Work out the finished part from the listing and answer in its coordinate system (mm). Face numbers are marked on the shaded views. A direction names the side the tool comes from. Give positions to 0.01 mm unless a question says otherwise; leave off trailing zeros. Write each loop counter-clockwise with the first axis right and the second up, starting at its lowest first coordinate (ties: lowest second). Pieces come first, ordered by that corner, then holes. Notation, with made-up numbers: (3, 21) -> (27, 21) arc R10 ccw to (27, 36) -> close; hole circle Ø6 at (87, -38.75). An arc over 180 degrees is marked (long way). Use a Markdown table: item, result. Add a question column.
Q1. Section A-A, the plane y = 7 is taken. Give the vertices of the cut face in (x, z).
Q2. Section D-D, the plane y = 1 is taken. Give the vertices of the cut face in (x, z).
Q3. For the marked faces 1, 2 and 3, determine the directions among +Z, -Z, +X, -X, +Y, -Y from which every point of the face is accessible in a straight line to the end or side of a thin tool.
Q4. Section C-C, the plane x = 13.35 is taken. Give the vertices of the cut face in (y, z).
Q5. Section B-B, the plane z = -5 is taken. Give the vertices of the cut face in (x, y), plus the area to 3 significant figures.
Q6. Each of these flat-tipped pins is pushed along its axis until it touches: pin 1 Ø2 at (x, z) = (1.5, -6) entering from -Y; pin 2 Ø1.4 at (y, z) = (4.5, 5.5) entering from +X; pin 3 Ø6 at (x, z) = (9.5, -0.5) entering from +Y. Where does it stop, or does it pass through?
Q7. For a pull along Z with two mould halves and no side action, classify the marked faces 4, 5 and 6 as pulls with the +Z half, pulls with the -Z half, needs draft (parallel to the pull), parting line crosses it, or undercut.
Q8. Consider line 1 (X direction, y = 0.3, z = 0); line 2 (Z direction, x = -13.35, y = 0.3); line 3 (X direction, y = 7.25, z = 6.5). Determine where each line is inside the solid, lowest interval first.
from build123d import *

# Parameters (mm, degrees)
SKETCH1_W                = 14.7
SKETCH1_H                = 15
BOSS_EXTRUDE1_DEPTH      = 15.4
SKETCH2_W                = 10.7
SKETCH2_H                = 14.684086862
CUT_EXTRUDE1_DEPTH       = 13
SKETCH4_W                = 2.7
SKETCH4_H                = 3.8
BOSS_EXTRUDE2_DEPTH      = 3
SKETCH5_W                = 10
SKETCH5_H                = 13.4
CUT_EXTRUDE2_DEPTH       = 23.572106681
SKETCH6_W                = 9.3
SKETCH6_H                = 3.8
SKETCH6_H_2              = 2.4
CUT_EXTRUDE3_DEPTH       = 23.719650085
BOSS_EXTRUDE3_DEPTH      = 12
BOSS_EXTRUDE3_DEPTH_BACK = 2.7
SKETCH7_W                = 15
SKETCH7_H                = 2
BOSS_EXTRUDE4_DEPTH      = 12
BOSS_EXTRUDE4_DEPTH_BACK = 2.7
SKETCH8_W                = 15
SKETCH8_H                = 2


with BuildPart() as part:
    # Sketch1 → Boss-Extrude1 (new body)
    with BuildSketch(Plane(origin=(0, 0, 0), x_dir=(1, 0, 0), z_dir=(0, 1, 0))):
        Rectangle(SKETCH1_W, SKETCH1_H)
    extrude(amount=BOSS_EXTRUDE1_DEPTH)

    # Sketch2 → Cut-Extrude1 (cut)
    with BuildSketch(Plane.XY.offset(7.5)):
        with Locations((0, 6.057956569)):
            Rectangle(SKETCH2_W, SKETCH2_H)
    extrude(amount=-CUT_EXTRUDE1_DEPTH, mode=Mode.SUBTRACT)

    # Sketch4 → Boss-Extrude2 (add)
    with BuildSketch(Plane.XY.offset(7.5)):
        with Locations((-6, 7.4)):
            Rectangle(SKETCH4_W, SKETCH4_H)
        with Locations((-6, 12.9)):
            Rectangle(SKETCH4_W, SKETCH4_H)
        with Locations((6, 12.9)):
            Rectangle(SKETCH4_W, SKETCH4_H)
        with Locations((6, 7.4)):
            Rectangle(SKETCH4_W, SKETCH4_H)
        with Locations((-6, 1.9)):
            Rectangle(SKETCH4_W, SKETCH4_H)
        with Locations((6, 1.9)):
            Rectangle(SKETCH4_W, SKETCH4_H)
    extrude(amount=-BOSS_EXTRUDE2_DEPTH)

    # Sketch5 → Cut-Extrude2 (cut, through all)
    with BuildSketch(Plane(origin=(7.35, 0, 0), x_dir=(0, 0, -1), z_dir=(1, 0, 0))):
        with Locations((0.5, 8.7)):
            Rectangle(SKETCH5_W, SKETCH5_H)
    extrude(amount=-CUT_EXTRUDE2_DEPTH, mode=Mode.SUBTRACT)

    # Sketch6 → Cut-Extrude3 (cut, through all)
    with BuildSketch(Plane.XY.offset(7.5)):
        with Locations((0, 7.4)):
            Rectangle(SKETCH6_W, SKETCH6_H)
        with Locations((0, 1.9)):
            Rectangle(SKETCH6_W, SKETCH6_H)
        with Locations((0, 12.2)):
            Rectangle(SKETCH6_W, SKETCH6_H_2)
    extrude(amount=-CUT_EXTRUDE3_DEPTH, mode=Mode.SUBTRACT)

    # Sketch7 → Boss-Extrude3 (add, two sides: drawn at the far end of the back side and taken through both)
    with BuildSketch(Plane.ZY.offset(7.35).offset(-BOSS_EXTRUDE3_DEPTH_BACK)):
        with Locations((0, 1)):
            Rectangle(SKETCH7_W, SKETCH7_H)
    extrude(amount=BOSS_EXTRUDE3_DEPTH + BOSS_EXTRUDE3_DEPTH_BACK)

    # Sketch8 → Boss-Extrude4 (add, two sides: drawn at the far end of the back side and taken through both)
    with BuildSketch(Plane(origin=(7.35, 0, 0), x_dir=(0, 0, -1), z_dir=(1, 0, 0)).offset(-BOSS_EXTRUDE4_DEPTH_BACK)):
        with Locations((0, 1)):
            Rectangle(SKETCH8_W, SKETCH8_H)
    extrude(amount=BOSS_EXTRUDE4_DEPTH + BOSS_EXTRUDE4_DEPTH_BACK)

    # Sketch10 → CSK for M3 Flat Head Machine Screw1 (revolve, cut)
    with BuildSketch(Plane(origin=(-13.35, 2, 0), x_dir=(0, 0, 1), z_dir=(1, 0, 0))):
        Polygon((0, 0), (0, 2), (1.7, 2), (1.7, 1.45), (3.15, 0), align=None)
    revolve(axis=Axis((-13.35, 8.35, 0), (0, -1, 0)), mode=Mode.SUBTRACT)

    # Sketch12 → CSK for M3 Flat Head Machine Screw2 (revolve, cut)
    with BuildSketch(Plane(origin=(13.35, 2, 0), x_dir=(0, 0, 1), z_dir=(1, 0, 0))):
        Polygon((0, 0), (0, 2), (1.7, 2), (1.7, 1.45), (3.15, 0), align=None)
    revolve(axis=Axis((13.35, 8.35, 0), (0, -1, 0)), mode=Mode.SUBTRACT)


solid = part.part
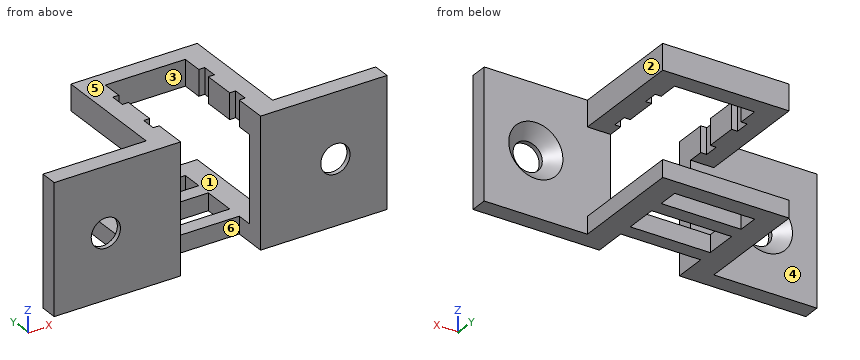
Result set:
| question | item | result |
|---|---|---|
| 1 | outline | (-7.35, -7.5) -> (-4.65, -7.5) -> (-4.65, -5.5) -> (-7.35, -5.5) -> close; (-7.35, 4.5) -> (-4.65, 4.5) -> (-4.65, 7.5) -> (-7.35, 7.5) -> close; (4.65, -7.5) -> (7.35, -7.5) -> (7.35, -5.5) -> (4.65, -5.5) -> close; (4.65, 4.5) -> (7.35, 4.5) -> (7.35, 7.5) -> (4.65, 7.5) -> close |
| 2 | outline | (-19.35, -7.5) -> (-4.65, -7.5) -> (-4.65, 7.5) -> (-19.35, 7.5) -> close; (4.65, -7.5) -> (19.35, -7.5) -> (19.35, 7.5) -> (4.65, 7.5) -> close; hole circle Ø4.3 at (-13.35, 0); hole circle Ø4.3 at (13.35, 0) |
| 3 | face 1 | +X, -X, +Y |
| 3 | face 2 | +Z, -Z, +X, +Y |
| 3 | face 3 | +Z, -Z, -Y |
| 4 | outline | (0, -7.5) -> (2, -7.5) -> (2, -3.15) -> (0.55, -1.7) -> (0, -1.7) -> close; (0, 1.7) -> (0.55, 1.7) -> (2, 3.15) -> (2, 7.5) -> (0, 7.5) -> close |
| 5 | outline | (-19.35, 0) -> (-4.65, 0) -> (-4.65, 2) -> (-19.35, 2) -> close; (4.65, 0) -> (19.35, 0) -> (19.35, 2) -> (4.65, 2) -> close |
| 5 | area | 58.8 mm2 |
| 6 | pin 1 | stops at y = 3.8 |
| 6 | pin 2 | stops at x = 7.35 |
| 6 | pin 3 | stops at y = 2 |
| 7 | face 4 | undercut |
| 7 | face 5 | pulls with the +Z half |
| 7 | face 6 | needs draft |
| 8 | line 1 | x = -19.35 to -15.05, -11.65 to -4.65, 4.65 to 11.65, 15.05 to 19.35 |
| 8 | line 2 | z = -7.5 to -1.7, 1.7 to 7.5 |
| 8 | line 3 | x = -7.35 to -4.65, 4.65 to 7.35 |
